The model under review builds one solid part; all positions refer to its coordinate system, in mm. A direction names the side the tool comes from. Give positions to 0.01 mm unless a question says otherwise; leave off trailing zeros. Order: outer loops, then holes, each group sorted by start corner. A loop starts at its lowest first (then second) coordinate and runs counter-clockwise, first axis right, second up. Notation, with made-up numbers: (-20.5, -19) - (26.5, -19) arc R19 cw to (26.5, -1) - close; hole circle Ø2 at (65, -20). An arc over 180 degrees is marked (long way). Write item = value, one per line. Start each with the question number.
1. We need section B-B, the plane y = -29. Give the boundary of the cut face in (x, z), and give its area (3 significant figures).
2. Machinability: for faces 1 (the flat face through (32.5, 6, 36)), 2 (the flat face through (-1, 4, 0)), 3 (the flat face through (-34.5, -54, 35)), 4 (the flat face through (-1, 114, 12)), 5 (the flat face through (-33.5, -59, 36)), which of the approach directions +Z, -Z, +X, -X, +Y, -Y give a long, thin tool a straight path to every point of the face, cutting with its end or side? Answer none if there is none.
3. Wall thickness on probe 1 along Z at (x, y) = (15.5, 59); probe 2 along X at (y, z) = (-46, 40); probe 3 along X at (y, z) = (-10.5, 27.5): over which ranges is each line inside the solid? List them lowest first.
4. We need section D-D, the plane y = 106.5. Give the boundary of the cut face in (x, z).
5. We need section A-A, the plane z = 32.5. Give the boundary of the cut face in (x, y).
6. For P1, Ø19.5, axis at y = -66.5, z = 43, coming from the +X side; P2, Ø1, axis at x = 26, y = -31, coming from the +Z side; P3, Ø1.1, axis at x = -34, z = 35.5, coming from the +Y side, all flat-tipped, find the tip position at first contact; note any pin that passes through.
7. We need section C-C, the plane x = 8. Give the boundary of the cut face in (y, z), and give its area (3 significant figures).
from build123d import *

# Parameters (mm, degrees)
F0_W     = 68
F0_H     = 188
F1_DEPTH = 1
F0_H_2   = 35
F2_DEPTH = 13
F3_W     = 68
F3_H     = 34
F4_DEPTH = 12
F5_W     = 65
F5_H     = 69
F6_DEPTH = 1
F7_W     = 65
F7_H     = 69
F8_DEPTH = 1


# Not quite as in the source:
# - a feature names something its author has since deleted; it is built from what else it names


with BuildPart() as f1:
    # F0 (on Top) → F1 (new body)
    with BuildSketch(Plane.XY):
        with Locations((145.9408301511, 2.5440129265)):
            Rectangle(F0_W, F0_H)
    extrude(amount=F1_DEPTH)

    # F0 (on Top) → F2 (join)
    with BuildSketch(Plane.XY):
        with Locations((145.9408301511, 114.0440129265)):
            Rectangle(F0_W, F0_H_2)
    extrude(amount=F2_DEPTH)

    # F3 (on face) → F4 (cut)
    with BuildSketch(Plane(origin=(0, 0, 0), x_dir=(1, 0, 0), z_dir=(0, 0, -1))):
        with Locations((145.9408301511, -114.5440129265)):
            Rectangle(F3_W, F3_H)
    extrude(amount=-F4_DEPTH, mode=Mode.SUBTRACT)

    # F5 (on face) → F6 (join)
    with BuildSketch(Plane.YZ.offset(179.9408301511)):
        with Locations((6.0440129265, 35.5)):
            Rectangle(F5_W, F5_H)
    extrude(amount=-F6_DEPTH)

    # F7 (on face) → F8 (join)
    with BuildSketch(Plane(origin=(111.9408301511, 0, 0), x_dir=(0, -1, 0), z_dir=(-1, 0, 0))):
        with Locations((58.9559870735, 35.5)):
            Rectangle(F7_W, F7_H)
    extrude(amount=-F8_DEPTH)


with BuildPart() as f1_1:
    # F9: moved
    add(f1.part.moved(Location((-146.441, 0, 0))))


solid = f1_1.part
Model answer:
q1.outline = (-34.5, 0) - (33.5, 0) - (33.5, 1) - (-33.5, 1) - (-33.5, 70) - (-34.5, 70) - close
q1.area = 137 mm2
q2.face_1 = +Z, -X, -Y
q2.face_2 = -Z, +X, -X, +Y, -Y
q2.face_3 = +Z, -Z, -X, +Y, -Y
q2.face_4 = -Z, +X, -X, +Y
q2.face_5 = +Z, +X, -Y
q3.probe_1 = 0 to 1
q3.probe_2 = -34.5 to -33.5
q3.probe_3 = 32.5 to 33.5
q4.outline = (-34.5, 12) - (33.5, 12) - (33.5, 13) - (-34.5, 13) - close
q5.outline = (-34.5, -91.46) - (-33.5, -91.46) - (-33.5, -26.46) - (-34.5, -26.46) - close; (32.5, -26.46) - (33.5, -26.46) - (33.5, 38.54) - (32.5, 38.54) - close
q6.P1 = -33.5
q6.P2 = 1
q6.P3 = -26.46
q7.outline = (-91.46, 0) - (97.54, 0) - (97.54, 12) - (131.54, 12) - (131.54, 13) - (96.54, 13) - (96.54, 1) - (-91.46, 1) - close
q7.area = 235 mm2
